```python
from build123d import *

# Parameters (mm, degrees)
ESQUISSE1_R             = 17
ESQUISSE1_R_2           = 14
ESQUISSE3_W             = 65
ESQUISSE3_H             = 45
ESQUISSE3_R             = 14
ESQUISSE3_R_2           = 2
BOSS_EXTRU_1_DEPTH      = 3
ESQUISSE4_W             = 56.431647226
ESQUISSE4_H             = 36.329386627
ENL_V_MAT_EXTRU_1_DEPTH = 10


with BuildPart() as part:
    # Balayage1: sweep along a path in Esquisse2
    with BuildLine(Plane(origin=(0, 0, 0), x_dir=(0, 0, -1), z_dir=(1, 0, 0))) as balayage1_path:
        ThreePointArc((0, 0), (42.265649833, -21.177861693), (60, -65))
    # Esquisse1 → Balayage1 (sweep)
    with BuildSketch(Plane.XY):
        Circle(ESQUISSE1_R)
        Circle(ESQUISSE1_R_2, mode=Mode.SUBTRACT)
    sweep(path=balayage1_path.line)

    # Esquisse3 → Boss.-Extru.1 (add)
    with BuildSketch(Plane.XY):
        Rectangle(ESQUISSE3_W, ESQUISSE3_H)
        Circle(ESQUISSE3_R, mode=Mode.SUBTRACT)
        with Locations((-23.25, 11.25)):
            Circle(ESQUISSE3_R_2, mode=Mode.SUBTRACT)
        with Locations((-23.25, -11.25)):
            Circle(ESQUISSE3_R_2, mode=Mode.SUBTRACT)
        with Locations((23.25, -11.25)):
            Circle(ESQUISSE3_R_2, mode=Mode.SUBTRACT)
        with Locations((23.25, 11.25)):
            Circle(ESQUISSE3_R_2, mode=Mode.SUBTRACT)
    extrude(amount=BOSS_EXTRU_1_DEPTH)

    # Esquisse4 → Enlèv. mat.-Extru.1 (cut)
    with BuildSketch(Plane(origin=(0, -63, 0), x_dir=(1, 0, 0), z_dir=(0, 1, 0))):
        with Locations((0, 60.039216013)):
            Rectangle(ESQUISSE4_W, ESQUISSE4_H)
    extrude(amount=-ENL_V_MAT_EXTRU_1_DEPTH, mode=Mode.SUBTRACT)


solid = part.part
```
Model file for the job. Use its own axes, mm. A direction names the side the tool comes from. Coordinates: 2 decimals unless noted, no trailing zeros. Order: outer loops, then holes, each group sorted by start corner. A loop starts at its lowest first (then second) coordinate and runs counter-clockwise, first axis right, second up. Notation, with made-up numbers: (-2, -12) -> (50, -12) arc R11 cw to (50, 1) -> close; hole circle Ø5 at (22.25, 10). An arc over 180 degrees is marked (long way). Answer as a JSON object with one key per item and string values. Group by question number.
1) Which spindle directions (+Z, -Z, +X, -X, +Y, -Y) get a long thin tool onto all of the face, cutting with end or side? Do faces 1 (the face through (14, 10, 0)), 2 (the face through (12.932, -5.362, 1.479)), 3 (the face through (0, 22.5, 1)). Say none if no direction does.
2) Pull direction X, two halves, no side cores. Call faces 4 (the face through (0, -22.5, 1)), 5 (the face through (-24.724, -9.898, 1.479)), 6 (the face through (-32.5, 0, 1)): +X half, -X half, draft (parallel to the pull), parting line (faces both ways), or undercut.
3) Cut at A-A, the plane x = 23.25. Write the cut outline in (y, z).
4) Cut at B-B, the plane y = -11.25. Count the separate pieces of the cut face and the enclosed holes in it, then the cut area to 3 significant figures.
5) Cut at C-C, the plane x = -29. Write the cut outline in (y, z), then the cut area to 3 significant figures.
6) Drill centre lines: L1, parallel to Y at x = -23, z = 1; L2, parallel to Z at x = 5, y = -21.5; L3, parallel to X at y = 0, z = 0.75. Where is each one in solid material? Low to high.
7) Flat gauge pins, fed straight in: pin 1 (4 mm diameter, centred on y = -14.5, z = -29.5, fed in from -X); pin 2 (25 mm diameter, centred on x = 0, y = 0, fed in from -Z); pin 3 (3 mm diameter, centred on x = -1, z = -66, fed in from +Y). Where does each tip first touch, or does it go through?
Check values:
{
 "1": {"face 1": "none", "face 2": "+Z", "face 3": "+Z, -Z, +X, -X, +Y"},
 "2": {"face 4": "draft", "face 5": "undercut", "face 6": "-X half"},
 "3": {"outline": "(-22.5, 0) -> (-13.25, 0) -> (-13.25, 3) -> (-22.5, 3) -> close; (-9.25, 0) -> (9.25, 0) -> (9.25, 3) -> (-9.25, 3) -> close; (13.25, 0) -> (22.5, 0) -> (22.5, 3) -> (13.25, 3) -> close"},
 "4": {"separate pieces": "3", "enclosed holes": "0", "area": "550 mm²"},
 "5": {"outline": "(-22.5, 0) -> (22.5, 0) -> (22.5, 3) -> (-22.5, 3) -> close", "area": "135 mm²"},
 "6": {"L1": "y = -22.5 to -13.23, -9.27 to 9.27, 13.23 to 22.5", "L2": "z = -62.91 to -59.12, -22.71 to -16.51, 0 to 3", "L3": "x = -32.5 to -14, 14 to 32.5"},
 "7": {"pin 1": "stops at x = -16.94", "pin 2": "stops at z = -57.18", "pin 3": "stops at y = -22.67"}
}
